from build123d import *

# Parameters (mm, degrees)
BOSS_EXTRUDE1_DEPTH = 1
SKETCH2_R           = 0.6
CUT_EXTRUDE1_DEPTH  = 10.861161189


with BuildPart() as part:
    # Sketch1 → Boss-Extrude1 (new body)
    with BuildSketch(Plane.XY):
        with BuildLine():
            Line((-3.8, -4.157546152), (-3.8, -7.3))
            ThreePointArc((-3.8, -7.3), (-3.653553391, -7.653553391), (-3.3, -7.8))
            Line((-3.3, -7.8), (-0.15, -7.8))
            Line((-0.15, -7.8), (-0.15, -4.797655678))
            ThreePointArc((-0.15, -4.797655678), (0, 4.8), (0.15, -4.797655678))
            Line((0.15, -4.797655678), (0.15, -7.8))
            Line((0.15, -7.8), (3.3, -7.8))
            ThreePointArc((3.3, -7.8), (3.653553391, -7.653553391), (3.8, -7.3))
            Line((3.8, -7.3), (3.8, -4.157546152))
            ThreePointArc((3.8, -4.157546152), (3.843564535, -3.953422006), (3.966666667, -3.784868155))
            ThreePointArc((3.966666667, -3.784868155), (0, 6.6), (-3.966666667, -3.784868155))
            ThreePointArc((-3.966666667, -3.784868155), (-3.843564535, -3.953422006), (-3.8, -4.157546152))
        make_face()
    extrude(amount=-BOSS_EXTRUDE1_DEPTH)

    # Sketch2 → Cut-Extrude1 (cut, through all)
    with BuildSketch(Plane.XY):
        with Locations((-2.15, -6.3)):
            Circle(SKETCH2_R)
        with Locations((2.15, -6.3)):
            Circle(SKETCH2_R)
    extrude(amount=-CUT_EXTRUDE1_DEPTH, mode=Mode.SUBTRACT)


solid = part.part
Read the model definition and answer for the solid it produces. Units are mm, in the model's axes. A direction names the side the tool comes from. Give positions to 0.01 mm unless a question says otherwise; leave off trailing zeros. Write each loop counter-clockwise with the first axis right and the second up, starting at its lowest first coordinate (ties: lowest second). Pieces come first, ordered by that corner, then holes. Notation, with made-up numbers: (44, 40) - (61, 40) arc R19 cw to (61, 52) - close; hole circle Ø9 at (6, -8). An arc over 180 degrees is marked (long way). Answer in a Markdown table with one row per item. Add a question column.
Item 1: Find the intervals of material crossed by L1, parallel to Y at x = -2.15, z = -0.45; L2, parallel to Y at x = 2, z = -0.9; L3, parallel to Y at x = 0, z = -0.7, in increasing order.
Item 2: Section C-C, the plane z = -0.35 is taken. Write down the section's boundary in (x, y).
Item 3: Section A-A, the plane y = -5.25 is taken. Write down the section's boundary in (x, z), and give its area (3 significant figures).
Item 4: Section B-B, the plane x = -3 is taken. Write down the section's boundary in (y, z), and give its area (3 significant figures).
Item 5: Section D-D, the plane x = 2 is taken. Write down the section's boundary in (y, z).
Item 6: Determine the mould class of faces 6 (the face through (2.072, -5.705, -0.493)), 7 (the face through (0.201, 6.597, -0.493)), 8 (the face through (-0.15, -6.3, -0.5)) for opening direction Y: pulls with the +Y half, pulls with the -Y half, needs draft (parallel to the pull), parting line crosses it, or undercut.
Item 7: A tool of negligible diameter and unlimited length cuts with its end or side. For faces 1 (the face through (3.8, -5.8, -0.5)), 2 (the face through (-2.228, -5.705, -0.493)), 3 (the face through (0.15, -6.3, -0.5)), 4 (the face through (-3.8, -5.7, -0.5)), 5 (the face through (1.7, -7.8, -0.5)), from which of +Z, -Z, +X, -X, +Y, -Y can it reach the whole face along a straight path? Write none if from no direction.
Item 8: A flat-ended cylindrical pin translates along its axis: P1, Ø0.5, axis at y = -6, z = -0.5, coming from the +X side. Find the tip coordinate at first contact, or state that the pin passes through.
Recorded:
| question | item | result |
|---|---|---|
| 1 | L1 | y = -7.8 to -6.9, -5.7 to -4.29, 4.29 to 6.2 |
| 1 | L2 | y = -7.8 to -6.88, -5.72 to -4.36, 4.36 to 6.25 |
| 1 | L3 | y = 4.8 to 6.6 |
| 2 | outline | (-3.97, -3.78) arc R0.5 cw to (-3.8, -4.16) - (-3.8, -7.3) arc R0.5 ccw to (-3.3, -7.8) - (-0.15, -7.8) - (-0.15, -4.8) arc R4.8 cw (long way) to (0.15, -4.8) - (0.15, -7.8) - (3.3, -7.8) arc R0.5 ccw to (3.8, -7.3) - (3.8, -4.16) arc R0.5 cw to (3.97, -3.78) arc R5.95 ccw (long way) to start; hole circle Ø1.2 at (-2.15, -6.3); hole circle Ø1.2 at (2.15, -6.3) |
| 3 | outline | (-3.8, -1) - (-0.15, -1) - (-0.15, 0) - (-3.8, 0) - close; (0.15, -1) - (3.8, -1) - (3.8, 0) - (0.15, 0) - close |
| 3 | area | 7.30 mm2 |
| 4 | outline | (-7.8, -1) - (-3.75, -1) - (-3.75, 0) - (-7.8, 0) - close; (3.75, -1) - (5.79, -1) - (5.79, 0) - (3.75, 0) - close |
| 4 | area | 6.09 mm2 |
| 5 | outline | (-7.8, -1) - (-6.88, -1) - (-6.88, 0) - (-7.8, 0) - close; (-5.72, -1) - (-4.36, -1) - (-4.36, 0) - (-5.72, 0) - close; (4.36, -1) - (6.25, -1) - (6.25, 0) - (4.36, 0) - close |
| 6 | face 6 | undercut |
| 6 | face 7 | parting line crosses it |
| 6 | face 8 | needs draft |
| 7 | face 1 | +Z, -Z, +X, -Y |
| 7 | face 2 | +Z, -Z |
| 7 | face 3 | +Z, -Z, -Y |
| 7 | face 4 | +Z, -Z, -X, -Y |
| 7 | face 5 | +Z, -Z, +X, -X, -Y |
| 8 | P1 | stops at x = 3.8 |
